Verification items for the finished model (mm, model axes). Face numbers are marked on the shaded views. A direction names the side the tool comes from. Give positions to 0.01 mm unless a question says otherwise; leave off trailing zeros. Loops run counter-clockwise (first coordinate to the right, second up) from the corner with the lowest first, then second, coordinate; pieces in that order, holes last. Notation, with made-up numbers: M -4,60 L 39,60 A8 ccw 39,74 Z; hole C 81.5,66.25 d5. An arc over 180 degrees is marked long. Use a Markdown table: item, result.
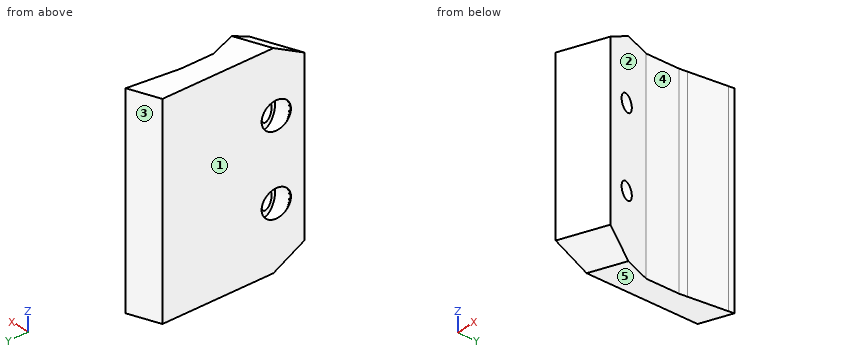
from build123d import *

# Parameters (mm, degrees)
EXTRUDE_1020_DEPTH     = 40.639999
CUT_EXTRUDE_START      = -9.474731536
CUT_EXTRUDE_1457_DEPTH = 9.474731536
SKETCH_5_6_R           = 1.631950308
EXTRUDE_1503_DEPTH     = 8.257914
CUT_EXTRUDE_2395_REACH = 52.464
SKETCH_11_R            = 2.75
CUT_EXTRUDE_2_REACH    = 52.464
SKETCH_18_R            = 2.75


# Read off the part's stored shape, not the designer's step: 切割边缘
with BuildPart() as part:
    # Sketch 255 → Extrude 1020 (new body)
    with BuildSketch(Plane.XY):
        Polygon((4.726521015, 20.743641369), (4.726521015, 19.19011116), (4.726521015, 14.125546455), (8.845423698, 3.395440102), (0, -5.59e-07), (0, 28.474460602), (5.956491721, 30.760943971), (5.827697754, 29.712001801), (4.915848732, 22.285591125), align=None)
    extrude(amount=EXTRUDE_1020_DEPTH)

    # Cut-Extrude 1457 outline → Cut-Extrude 1457 (cut)
    with BuildSketch(Plane(origin=(8.845423511, 3.395440589, 0), x_dir=(0, 0, -1), z_dir=(0.9335804043176853, 0.35836800732491086, 0)).offset(CUT_EXTRUDE_START)):
        Polygon((-37.293439923, -5.22e-07), (-40.63999939, 5.796406388), (-40.63999939, -5.22e-07), align=None)
    cut_extrude_1457 = extrude(amount=CUT_EXTRUDE_1457_DEPTH, mode=Mode.SUBTRACT)

    # 草图5<6> → Extrude 1503 (add)
    with BuildSketch(Plane(origin=(8.845423511, 3.395440589, 0), x_dir=(0, 0, -1), z_dir=(0.9335804043176853, 0.35836800732491086, 0))):
        with Locations(Location((-28.25750129, 5.25344969, 0), (0, 0, 90))):
            Circle(SKETCH_5_6_R)
    extrude_1503 = extrude(amount=-EXTRUDE_1503_DEPTH)

    # 镜向6: Cut-Extrude 1457, Extrude 1503 across plane
    add(cut_extrude_1457.mirror(Plane.XY.offset(20.319999695)), mode=Mode.SUBTRACT)
    add(extrude_1503.mirror(Plane.XY.offset(20.319999695)))

    # 草图10 → M2.5 凹头盖螺钉的柱形沉头孔2 (revolve, cut)
    with BuildSketch(Plane(origin=(-0.746671694, 5.340586006, 28.25750129), x_dir=(0.3583680073249109, -0.9335804043176852, 0), z_dir=(0, 0, 1))):
        Polygon((0, 0), (0, 18.064835324), (1.635, 18.064835324), (1.635, 2.5), (2.75, 2.5), (2.75, 0.025), (2.775, 0), align=None)
    revolve(axis=Axis((-6.674907261, 3.06494916, 28.25750129), (0.9335804043176852, 0.358368007324911, 0)), mode=Mode.SUBTRACT)

    # 草图11 → Cut-Extrude 2395 (cut, up to next)
    with BuildSketch(Plane(origin=(3.469947614, 1.331988339, 0), x_dir=(0, 0, 1), z_dir=(-0.9335804043176853, -0.3583680073249109, 0)), mode=Mode.PRIVATE) as cut_extrude_2395_sk1:
        with Locations(Location((28.25750129, 5.25344969, 0), (0, 0, 270))):
            Circle(SKETCH_11_R)
    cut_extrude_2395_tool1 = extrude(cut_extrude_2395_sk1.sketch, amount=CUT_EXTRUDE_2395_REACH, mode=Mode.PRIVATE) & part.part
    add(cut_extrude_2395_tool1.solids().sort_by_distance((1.587279, 6.236506, 28.257501))[0], mode=Mode.SUBTRACT)

    # 草图17 → M2.5 凹头盖螺钉的柱形沉头孔5 (revolve, cut)
    with BuildSketch(Plane(origin=(-0.746671694, 5.340586006, 12.3824981), x_dir=(0.3583680073249109, -0.9335804043176852, 0), z_dir=(0, 0, 1))):
        Polygon((0, 0), (0, 18.064835324), (1.635, 18.064835324), (1.635, 2.5), (2.75, 2.5), (2.75, 0.025), (2.775, 0), align=None)
    revolve(axis=Axis((-6.674907261, 3.06494916, 12.3824981), (0.9335804043176852, 0.358368007324911, 0)), mode=Mode.SUBTRACT)

    # 草图18 → 修整螺丝2 (cut, up to next)
    with BuildSketch(Plane(origin=(3.469947614, 1.331988339, 0), x_dir=(0, 0, 1), z_dir=(-0.9335804043176853, -0.3583680073249109, 0)), mode=Mode.PRIVATE) as cut_extrude_2_sk1:
        with Locations(Location((12.3824981, 5.25344969, 0), (0, 0, 270))):
            Circle(SKETCH_18_R)
    cut_extrude_2_tool1 = extrude(cut_extrude_2_sk1.sketch, amount=CUT_EXTRUDE_2_REACH, mode=Mode.PRIVATE) & part.part
    add(cut_extrude_2_tool1.solids().sort_by_distance((1.587279, 6.236506, 12.382498))[0], mode=Mode.SUBTRACT)


solid = part.part
(1) Cross-section at D-D on x = 8.25. Record the cut outline in (y, z), then the cut area to 3 significant figures.
Results below:
| item | result |
|---|---|
| outline | M 3.17,3.35 L 4.95,2.39 L 4.95,38.25 L 3.17,37.29 Z |
| area | 62.1 mm^2 |
(2) Cross-section at A-A on z = 19.5. Record the cut outline in (x, y).
Results below:
| item | result |
|---|---|
| outline | M 0,0 L 8.85,3.4 L 4.73,14.13 L 4.73,20.74 L 5.96,30.76 L 0,28.47 Z |
(3) Material ranges on line 1 (Z direction, x = 5.75, y = 9); line 2 (Z direction, x = 0.5, y = 4); line 3 (X direction, y = 13, z = 29), recorded low to high.
Results below:
| item | result |
|---|---|
| line 1 | 0 to 11.16, 13.6 to 27.04, 29.48 to 40.64 |
| line 2 | 1.29 to 10.22, 14.55 to 26.09, 30.42 to 39.35 |
| line 3 | 0 to 5.16 |
(4) Cross-section at B-B on x = 3.5. State how many separate pieces and enclosed holes the cut face has, then the cut area to 3 significant figures.
Results below:
| item | result |
|---|---|
| separate pieces | 1 |
| enclosed holes | 2 |
| area | 1,120 mm^2 |
(5) Set-up check for the marked faces 1 and 2: record each of +Z, -Z, +X, -X, +Y, -Y from which the full face is reachable in a straight line by a thin tool's end or side.
Results below:
| item | result |
|---|---|
| face 1 | +Z, -Z, -X, +Y, -Y |
| face 2 | +Z, -Z, +X |
(6) Cross-section at C-C on y = 2. Record the cut outline in (x, z).
Results below:
| item | result |
|---|---|
| outline | M 0,2.27 L 5.21,3.35 L 5.21,37.29 L 0,38.37 Z |
(7) Gauge pin test, flat ends, axial feed: P1, Ø4, axis at x = 4, y = 11.5, coming from the -Z side; P2, Ø1, axis at x = 4, z = 11, coming from the -Y side; P3, Ø3, axis at x = 6, z = 12, coming from the -Y side; P4, Ø8, axis at y = 18, z = 23.5, coming from the +X side. Record the tip position at first contact, or that the pin passes through.
Results below:
| item | result |
|---|---|
| P1 | z = 0 |
| P2 | y = 1.34 |
| P3 | y = 1.73 |
| P4 | x = 4.88 |
(8) Draft check along Y on the marked faces 3, 4 and 5. Enter one of: +Y half, -Y half, draft (parallel to the pull), parting line (faces both ways), or undercut.
Results below:
| item | result |
|---|---|
| face 3 | +Y half |
| face 4 | undercut |
| face 5 | draft |
